Design review of the part built by this model. Coordinates are the model's own, in mm. A direction names the side the tool comes from. Round coordinates to 2 decimals unless told otherwise and drop trailing zeros. Loops run counter-clockwise (first coordinate to the right, second up) from the corner with the lowest first, then second, coordinate; pieces in that order, holes last. Notation, with made-up numbers: (88.5, -14) - (114.5, -14) arc R20 cw to (114.5, 3) - close; hole circle Ø1 at (41.5, 6.5). An arc over 180 degrees is marked (long way). Return JSON: item names as keys, results as strings. Group by question number.
from build123d import *

# Parameters (mm, degrees)
SKETCH1_R           = 1.778
BOSS_EXTRUDE1_DEPTH = 3.175


with BuildPart() as part:
    # Sketch1 → Boss-Extrude1 (new body)
    with BuildSketch(Plane(origin=(0, 3.175, 0), x_dir=(1, 0, 0), z_dir=(0, 1, 0))):
        with BuildLine():
            Line((4.7625, 4.7625), (4.7625, 19.558))
            ThreePointArc((4.7625, 19.558), (0, 24.3205), (-4.7625, 19.558))
            Line((-4.7625, 19.558), (-4.7625, 4.7625))
            Line((-4.7625, 4.7625), (-9.779, 4.7625))
            ThreePointArc((-9.779, 4.7625), (-14.5415, 0), (-9.779, -4.7625))
            Line((-9.779, -4.7625), (9.779, -4.7625))
            ThreePointArc((9.779, -4.7625), (14.5415, 0), (9.779, 4.7625))
            Line((9.779, 4.7625), (4.7625, 4.7625))
        make_face()
        with Locations((0, 19.558)):
            Circle(SKETCH1_R, mode=Mode.SUBTRACT)
        with Locations((9.779, 0)):
            Circle(SKETCH1_R, mode=Mode.SUBTRACT)
        with Locations((0, 9.779)):
            Circle(SKETCH1_R, mode=Mode.SUBTRACT)
        with Locations((-9.779, 0)):
            Circle(SKETCH1_R, mode=Mode.SUBTRACT)
        Circle(SKETCH1_R, mode=Mode.SUBTRACT)
    extrude(amount=-BOSS_EXTRUDE1_DEPTH)


solid = part.part
Q1. Add section D-D, the plane x = 7.5. State the section outline as (y, z) points (1 decimal).
Q2. For line 1 (Z direction, x = 0, y = 0.85); line 2 (X direction, y = 1.1, z = 0); line 3 (Z direction, x = 1, y = 2.35), list the stretches that pass through material, from the lowest coordinate up.
Q3. Tool access review of faces 1 (the cylindrical face through (-0.385, 1.61, 1.736)), 2 (the flat face through (4.762, 2, -12)), 3 (the flat face through (-4.762, 2, -12)): name each direction out of +Z, -Z, +X, -X, +Y, -Y from which nothing blocks a thin tool from reaching the whole face with its end or side.
Q4. Add section C-C, the plane y = 0.6. State the section outline as (x, z) points (1 decimal), plus the area to 3 significant figures.
Q5. Draft analysis for pull direction X (two halves, no side actions). For faces 4 (the flat face through (-7, 2, -4.762)), 5 (the cylindrical face through (-14.54, 1.61, -0.1)), 6 (the cylindrical face through (-11.19, 1.61, 1.08)), state which applies: pulls with the +X half, pulls with the -X half, needs draft (parallel to the pull), parting line crosses it, or undercut.
Q6. Add section A-A, the plane x = 0. State the section outline as (y, z) points (1 decimal).
Q7. Add section B-B, the plane z = 0. State the section outline as (x, y) points (1 decimal), plus the area to 3 significant figures.
Q8. Insertion check: pin 1 Ø1.6 at (x, y) = (-8.5, 1.5) entering from -Z. The pin has a flat end and moves straight along its axis. Give the tip position at first contact, or say it passes through.
Evaluation:
{
 "1": {"outline": "(0, -4.8) - (3.2, -4.8) - (3.2, 4.8) - (0, 4.8) - close"},
 "2": {"line 1": "-24.32 to -21.34, -17.78 to -11.56, -8 to -1.78, 1.78 to 4.76", "line 2": "-14.54 to -11.56, -8 to -1.78, 1.78 to 8, 11.56 to 14.54", "line 3": "-24.21 to -21.03, -18.09 to -11.25, -8.31 to -1.47, 1.47 to 4.76"},
 "3": {"face 1": "+Y, -Y", "face 2": "-Z, +X, +Y, -Y", "face 3": "-Z, -X, +Y, -Y"},
 "4": {"outline": "(-9.8, -4.8) - (-4.8, -4.8) - (-4.8, -19.6) arc R4.8 ccw to (4.8, -19.6) - (4.8, -4.8) - (9.8, -4.8) arc R4.8 ccw to (9.8, 4.8) - (-9.8, 4.8) arc R4.8 ccw to start; hole circle Ø3.6 at (-9.8, 0); hole circle Ø3.6 at (0, -19.6); hole circle Ø3.6 at (0, -9.8); hole circle Ø3.6 at (0, 0); hole circle Ø3.6 at (9.8, 0)", "area": "384 mm²"},
 "5": {"face 4": "needs draft", "face 5": "pulls with the -X half", "face 6": "undercut"},
 "6": {"outline": "(0, -24.3) - (3.2, -24.3) - (3.2, -21.3) - (0, -21.3) - close; (0, -17.8) - (3.2, -17.8) - (3.2, -11.6) - (0, -11.6) - close; (0, -8) - (3.2, -8) - (3.2, -1.8) - (0, -1.8) - close; (0, 1.8) - (3.2, 1.8) - (3.2, 4.8) - (0, 4.8) - close"},
 "7": {"outline": "(-14.5, 0) - (-11.6, 0) - (-11.6, 3.2) - (-14.5, 3.2) - close; (-8, 0) - (-1.8, 0) - (-1.8, 3.2) - (-8, 3.2) - close; (1.8, 0) - (8, 0) - (8, 3.2) - (1.8, 3.2) - close; (11.6, 0) - (14.5, 0) - (14.5, 3.2) - (11.6, 3.2) - close", "area": "58.5 mm²"},
 "8": {"pin 1": "z = -4.76"}
}
